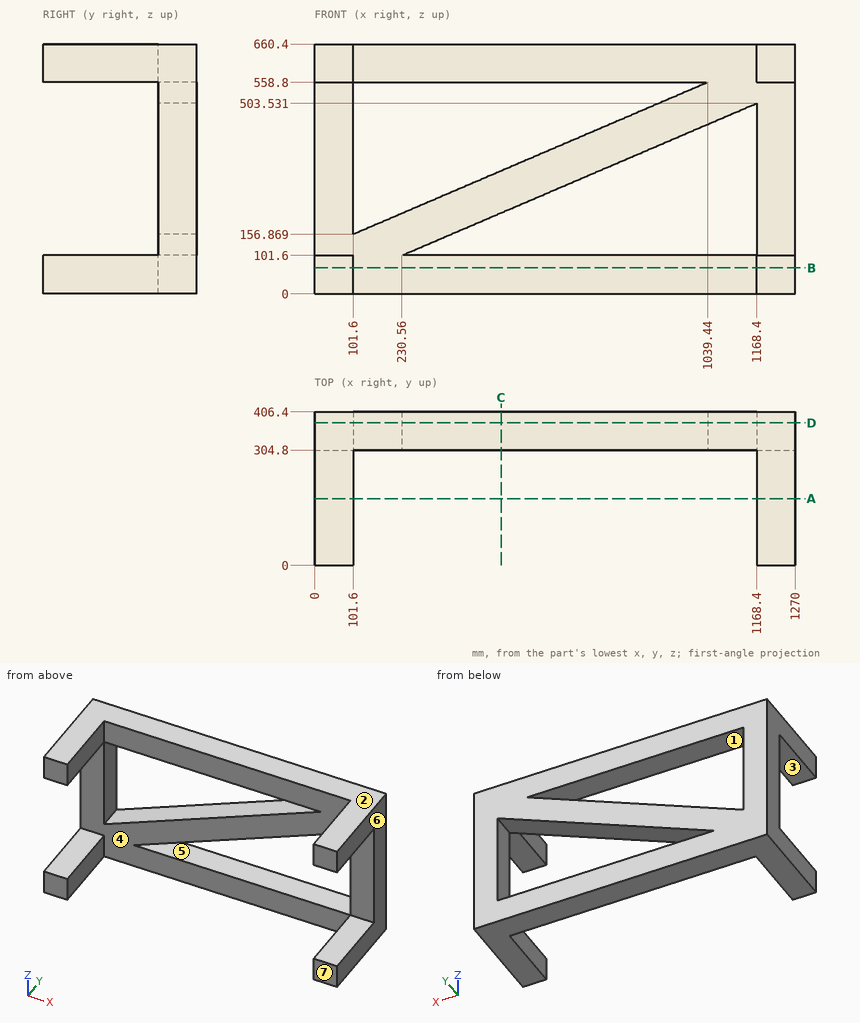
Print and shaded views of the part. All mm, measured from the part's lowest x, y and z. A direction names the side the tool comes from. Round coordinates to 2 decimals unless told otherwise and drop trailing zeros. Write each loop counter-clockwise with the first axis right and the second up, starting at its lowest first coordinate (ties: lowest second). Pieces come first, ordered by that corner, then holes. Notation, with made-up numbers: (0.25, 11.5) - (33.25, 11.5) arc R27 ccw to (33.25, 39.5) - close; hole circle Ø6 at (-33.5, -22). An arc over 180 degrees is marked (long way). Write each question's results on one line, items separated by ' | '. Start each with the question number.
Item 1: Mould opens along X. For the marked faces 4, 5, 6 and 7 say: pulls with the +X half, pulls with the -X half, needs draft (parallel to the pull), parting line crosses it, or undercut.
Item 2: Which spindle directions (+Z, -Z, +X, -X, +Y, -Y) get a long thin tool onto all of the face, cutting with end or side? Do the marked faces 1, 2 and 3. Say none if no direction does.
Item 3: Saw through at C-C (x = 493). Write the cut outline in (y, z), and give its area (3 significant figures).
Item 4: Saw through at D-D (y = 377). Write the cut outline in (x, z), and give its area (3 significant figures).
Item 5: Wall check: L1, parallel to X at y = 81.5, z = 566; L2, parallel to Z at x = 290, y = 383.5 (1 decimal); L3, parallel to Z at x = 1195.5, y = 87.5. Give the ranges that are in metal, low to high. Write a range as [from, to].
Item 6: Saw through at B-B (z = 68.5). Write the cut outline in (x, y).
Item 7: Saw through at A-A (y = 176.5). Write the cut outline in (x, z), and give its area (3 significant figures).
Results are:
1) face 4: undercut | face 5: undercut | face 6: pulls with the +X half | face 7: needs draft
2) face 1: +Y, -Y | face 2: +Z, +X, -X, +Y, -Y | face 3: +X, -X, -Y
3) outline: (304.8, 0) - (406.4, 0) - (406.4, 101.6) - (304.8, 101.6) - close; (304.8, 214.07) - (406.4, 214.07) - (406.4, 324.61) - (304.8, 324.61) - close; (304.8, 558.8) - (406.4, 558.8) - (406.4, 660.4) - (304.8, 660.4) - close | area: 31,900 mm²
4) outline: (0, 0) - (1270, 0) - (1270, 660.4) - (0, 660.4) - close; hole (101.6, 156.87) - (1039.44, 558.8) - (101.6, 558.8) - close; hole (230.56, 101.6) - (1168.4, 101.6) - (1168.4, 503.53) - close | area: 462,000 mm²
5) L1: x = [0, 101.6], [1168.4, 1270] | L2: z = [0, 101.6], [127.1, 237.6], [558.8, 660.4] | L3: z = [0, 101.6], [558.8, 660.4]
6) outline: (0, 0) - (101.6, 0) - (101.6, 304.8) - (1168.4, 304.8) - (1168.4, 0) - (1270, 0) - (1270, 406.4) - (0, 406.4) - close
7) outline: (0, 0) - (101.6, 0) - (101.6, 101.6) - (0, 101.6) - close; (0, 558.8) - (101.6, 558.8) - (101.6, 660.4) - (0, 660.4) - close; (1168.4, 0) - (1270, 0) - (1270, 101.6) - (1168.4, 101.6) - close; (1168.4, 558.8) - (1270, 558.8) - (1270, 660.4) - (1168.4, 660.4) - close | area: 41,300 mm²
